The model under review builds one solid part; all positions refer to its coordinate system, in mm. Give positions to 0.01 mm unless a question says otherwise; leave off trailing zeros. Write each loop counter-clockwise with the first axis right and the second up, starting at its lowest first coordinate (ties: lowest second). Pieces come first, ordered by that corner, then holes. Notation, with made-up numbers: (33, 82.25) - (52, 82.25) arc R30 cw to (52, 115.25) - close; hole circle Ø7 at (-28, 10.5). An arc over 180 degrees is marked (long way). Write item = value, one per line.
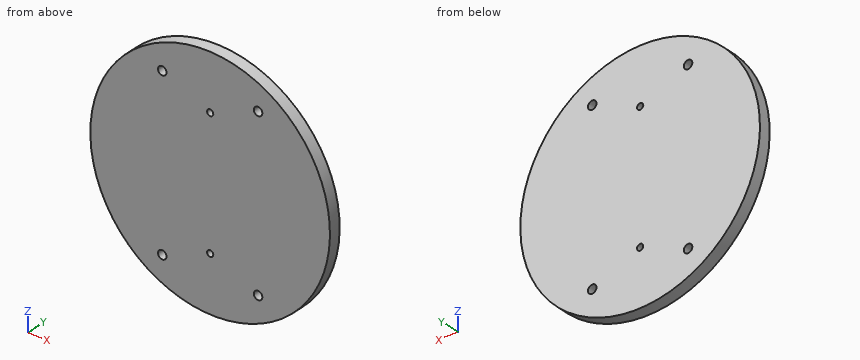
```python
from build123d import *

# Parameters (mm, degrees)
SKETCH1_R                   = 63.5
BOSS_EXTRUDE1_DEPTH         = 6.35
F_8_CLEARANCE_HOLE1_D       = 4.4958
TAP_DRILL_FOR_M4X0_7_TAP1_D = 3.3


with BuildPart() as part:
    # Sketch1 → Boss-Extrude1 (new body)
    with BuildSketch(Plane(origin=(0, 0, 0), x_dir=(1, 0, 0), z_dir=(0, 1, 0))):
        with Locations(Location((0, 0, 0), (0, 0, 270))):
            Circle(SKETCH1_R)
    extrude(amount=BOSS_EXTRUDE1_DEPTH)

    # #8 Clearance Hole1 (through all)
    with Locations(Plane(origin=(0, 6.35, 0), x_dir=(1, 0, 0), z_dir=(0, 1, 0))):
        with Locations((-25.4, -44.45), (25.4, -44.45), (25.4, 44.45), (-25.4, 44.45)):
            Hole(F_8_CLEARANCE_HOLE1_D / 2)

    # Tap Drill for M4x0.7 Tap1 (through all)
    with Locations(Plane(origin=(0, 6.35, 0), x_dir=(1, 0, 0), z_dir=(0, 1, 0))):
        with Locations((0, 34), (0, -34)):
            Hole(TAP_DRILL_FOR_M4X0_7_TAP1_D / 2)


solid = part.part
```
1. Take a section at A-A on x = 0. Give the boundary of the cut face in (y, z).
Findings below:
outline = (0, -63.5) - (6.35, -63.5) - (6.35, -35.65) - (0, -35.65) - close; (0, -32.35) - (6.35, -32.35) - (6.35, 32.35) - (0, 32.35) - close; (0, 35.65) - (6.35, 35.65) - (6.35, 63.5) - (0, 63.5) - close
2. Take a section at D-D on x = -25.4. Give the boundary of the cut face in (y, z), and give its area (3 significant figures).
Findings below:
outline = (0, -58.2) - (6.35, -58.2) - (6.35, -46.7) - (0, -46.7) - close; (0, -42.2) - (6.35, -42.2) - (6.35, 42.2) - (0, 42.2) - close; (0, 46.7) - (6.35, 46.7) - (6.35, 58.2) - (0, 58.2) - close
area = 682 mm²
3. Take a section at B-B on z = 34. Give the boundary of the cut face in (x, y), and give its area (3 significant figures).
Findings below:
outline = (-53.63, 0) - (-1.65, 0) - (-1.65, 6.35) - (-53.63, 6.35) - close; (1.65, 0) - (53.63, 0) - (53.63, 6.35) - (1.65, 6.35) - close
area = 660 mm²
4. Take a section at C-C on y = 2. Give the boundary of the cut face in (x, z), and give its area (3 significant figures).
Findings below:
outline = circle Ø127 at (0, 0); hole circle Ø4.5 at (-25.4, -44.45); hole circle Ø4.5 at (-25.4, 44.45); hole circle Ø3.3 at (0, -34); hole circle Ø3.3 at (0, 34); hole circle Ø4.5 at (25.4, -44.45); hole circle Ø4.5 at (25.4, 44.45)
area = 12,600 mm²
5. For line 1 (X direction, y = 1.75, z = -44.45); line 2 (Z direction, x = 25.4, y = 3.5); line 3 (X direction, y = 3, z = -34), list the stretches that pass through material, from the lowest coordinate up. Write a range as from..to.
Findings below:
line_1 = -45.35..-27.65, -23.15..23.15, 27.65..45.35
line_2 = -58.2..-46.7, -42.2..42.2, 46.7..58.2
line_3 = -53.63..-1.65, 1.65..53.63
6. Insertion check: P1, Ø1, axis at y = 1.5, z = -16.5, coming from the +X side; P2, Ø1, axis at x = -45.5, y = 2.5, coming from the +Z side; P3, Ø5, axis at x = -25.4, z = 44.45, coming from the -Y side; P4, Ø3, axis at x = 19.5, y = 3.5, coming from the +Z side. Each pin has a flat end and moves straight along its axis. Give the tip position at first contact, or say it passes through.
Findings below:
P1 = 61.45
P2 = 44.8
P3 = 0
P4 = 60.9
